Input: part model. Units: mm. Frame: model coordinates. A direction names the side the tool comes from. Round coordinates to 2 decimals unless told otherwise and drop trailing zeros. Loops run counter-clockwise (first coordinate to the right, second up) from the corner with the lowest first, then second, coordinate; pieces in that order, holes last. Notation, with made-up numbers: (-27.75, -28.5) -> (-3.75, -28.5) arc R33 cw to (-3.75, 7.5) -> close; hole circle Ø7 at (69, 74). An arc over 180 degrees is marked (long way). One line per question, with ' | ' between items. Start each with the question number.
Q1. Cut plane B-B on x = -32.5. Return loops of the section in (y, z).
Q2. Cut plane C-C on x = -21. Return loops of the section in (y, z).
Q3. Contact query for flat-ended pins moving along their axis: P1, Ø5.5, axis at x = -29.5, z = -3.5, coming from the +Y side; P2, Ø2.5, axis at x = -11, y = -3, coming from the +Z side; P3, Ø5, axis at x = -9, y = 1.5, coming from the -Z side. Output: stop coordinate, or through.
Q4. Mould query, pull axis Y, two halves, no side actions, for faces 4 (the face through (-6.23, 3.23, -4.55)), 5 (the face through (-47.17, -5.96, 0.02)), 6 (the face through (-47.728, 4.148, 4.897)). Classes: pulls with the +Y half, pulls with the -Y half, needs draft (parallel to the pull), parting line crosses it, or undercut.
Q5. Access query for faces 1 (the face through (-25, 10.058, 5)), 2 (the face through (-4.981, -2.624, -4.55)), 3 (the face through (-4.981, -2.624, 4.65)). Directions: +Z, -Z, +X, -X, +Y, -Y. A direction counts if a zero-diameter tool reaches every point of the face in a straight line with its end or side. Return the directions, or none.
Q6. Material intervals for L1, parallel to X at y = 5.5, z = 4; L2, parallel to X at y = 4.75, z = 5.75; L3, parallel to Z at x = -17, y = 10.5, sorted ascending.
Q7. Cut plane A-A on y = 4.75. Return loops of the section in (x, z), and give its area (3 significant figures).
from build123d import *

# Parameters (mm, degrees)
F1_DEPTH    = 8.2
F2_DEPTH    = 1
F4_DEPTH    = 5.5
F15_DEPTH   = 5.5
F5_R        = 2
F16_R       = 0.5
F17_R       = 2
F18_R       = 5
F19_R       = 0.5
F6_R        = 0.59999
F8_DEPTH    = 8.2
F9_T1_DEPTH = 31.0823571676
F10_R       = 4
F12_DEPTH   = 1.5
F13_R       = 7


# Not quite as in the source:
# - a fillet or chamfer that OpenCascade refuses, or shapes differently, is made with other operations: its cross-section is extruded or revolved along the edge and cut away or added
# - a fillet or chamfer is up to 0.001 mm smaller than in the source, because OpenCascade refuses the exact size


with BuildPart() as f1:
    # F0 (on Top) → F1 (new body, symmetric)
    with BuildSketch(Plane.XY):
        with BuildLine():
            Line((-7.6991717756, 9.5581562555), (-40.1991717756, 9.5581562555))
            ThreePointArc((-40.1991717756, 9.5581562555), (-47.4491717756, 2.3081562555), (-40.1991717756, -4.9418437445))
            ThreePointArc((-40.1991717756, -4.9418437445), (-38.6431985652, -1.6852820196), (-42.1543481568, -2.5207911129))
            ThreePointArc((-42.1543481568, -2.5207911129), (-44.8427156809, 2.8081562555), (-40.1991717756, 6.5581562555))
            Line((-40.1991717756, 6.5581562555), (-16.7462805126, 6.5581562555))
            Line((-16.7462805126, 6.5581562555), (-11.035484998, -2.9462035475))
            ThreePointArc((-11.035484998, -2.9462035475), (-4.6547300014, -4.5371044474), (-3.0638291014, 1.8436505492))
            Line((-3.0638291014, 1.8436505492), (-7.6991717756, 9.5581562555))
        make_face()
        with BuildLine():
            Line((-15.346320436, 6.5581562555), (-8.229856713, 6.5581562555))
            Line((-8.229856713, 6.5581562555), (-4.7781637028, 0.8135743994))
            ThreePointArc((-4.7781637028, 0.8135743994), (-5.8216578415, -3.3716519963), (-10.0068842371, -2.3281578576))
            Line((-10.0068842371, -2.3281578576), (-15.346320436, 6.5581562555))
        make_face(mode=Mode.SUBTRACT)
    extrude(amount=F1_DEPTH, both=True)

    # F0 (on Top) → F2 (join, symmetric)
    with BuildSketch(Plane.XY):
        with BuildLine():
            Line((-4.7781637028, 0.8135743994), (-8.229856713, 6.5581562555))
            Line((-8.229856713, 6.5581562555), (-15.346320436, 6.5581562555))
            Line((-15.346320436, 6.5581562555), (-10.0068842371, -2.3281578576))
            ThreePointArc((-10.0068842371, -2.3281578576), (-5.8216578415, -3.3716519963), (-4.7781637028, 0.8135743994))
        make_face()
    extrude(amount=F2_DEPTH, both=True)

    # F3 (on face) → F4 (cut)
    with BuildSketch(Plane.XY.offset(8.2)):
        Polygon((-9.8084988335, -7.0643632576), (-7.0496570497, -0.5512764992), (-8.3826289276, 1.6671612479), (-13.2850058391, -1.2784839779), align=None)
    extrude(amount=-F4_DEPTH, mode=Mode.SUBTRACT)

    # F14 (on face) → F15 (cut)
    with BuildSketch(Plane(origin=(0, 0, -8.2), x_dir=(1, 0, 0), z_dir=(0, 0, -1))):
        with BuildLine():
            Line((-12.3684568759, 0.7277658005), (-11.3398561151, 0.1097201106))
            Line((-11.3398561151, 0.1097201106), (-10.0068842371, 2.3281578576))
            ThreePointArc((-10.0068842371, 2.3281578576), (-9.3022346771, 3.1354223006), (-8.3618696665, 3.649154264))
            Line((-8.3618696665, 3.649154264), (-8.8633257373, 4.8329941325))
            ThreePointArc((-8.8633257373, 4.8329941325), (-10.099006978, 4.0618270279), (-11.035484998, 2.9462035475))
            Line((-11.035484998, 2.9462035475), (-12.3684568759, 0.7277658005))
        make_face()
    extrude(amount=-F15_DEPTH, mode=Mode.SUBTRACT)

    # F5
    f5_edges = [f1.edges().sort_by_distance(p)[0] for p in [
        (-16.746281, 6.558156, 0),
    ]]
    fillet(f5_edges, radius=F5_R)

    # F16
    f16_edges = [f1.edges().sort_by_distance(p)[0] for p in [
        (-15.34632, 6.558156, -4.6),
        (-15.34632, 6.558156, 4.6),
    ]]
    fillet(f16_edges, radius=F16_R)

    # F17
    f17_edges = [f1.edges().sort_by_distance(p)[0] for p in [
        (-8.229857, 6.558156, -4.6),
        (-8.229857, 6.558156, 4.6),
    ]]
    fillet(f17_edges, radius=F17_R)

    # F18
    f18_edges = [f1.edges().sort_by_distance(p)[0] for p in [
        (-7.699172, 9.558156, 0),
    ]]
    fillet(f18_edges, radius=F18_R)

    # F19
    f19_edges = [f1.edges().sort_by_distance(p)[0] for p in [
        (-42.154348, -2.520791, 0),
    ]]
    fillet(f19_edges, radius=F19_R)

    # F6 (radius 0.6 in the source; OpenCascade refuses exactly that, so slightly less here)
    f6_edges = [f1.edges().sort_by_distance(p)[0] for p in [
        (-12.368457, -0.727766, 5.45),
        (-11.339856, -0.10972, 5.45),
        (-8.36187, -3.649154, 5.45),
        (-8.863326, -4.832994, 5.45),
        (-8.863326, -4.832994, -5.45),
        (-8.36187, -3.649154, -5.45),
        (-12.368457, -0.727766, -5.45),
        (-11.339856, -0.10972, -5.45),
    ]]
    fillet(f6_edges, radius=F6_R)

    # F7 (on Top) → F8 (join, symmetric)
    with BuildSketch(Plane.XY):
        with BuildLine():
            ThreePointArc((-40.1991717756, -4.9418437445), (-47.4491717756, 2.3081562555), (-40.1991717756, 9.5581562555))
            Line((-40.1991717756, 9.5581562555), (-10.5280356666, 9.5581562555))
            ThreePointArc((-10.5280356666, 9.5581562555), (-8.065917866, 8.9099347352), (-6.242199163, 7.13334663))
            Line((-6.242199163, 7.13334663), (-3.0638291014, 1.8436505492))
            ThreePointArc((-3.0638291014, 1.8436505492), (-3.0131583432, -2.8597777863), (-7.0927569488, -5.2010767528))
            Line((-7.0927569488, -5.2010767528), (-4.8792576743, -5.2215941063))
            ThreePointArc((-4.8792576743, -5.2215941063), (-2.1256697511, -2.0601996528), (-2.6352454511, 2.1011695866))
            Line((-2.6352454511, 2.1011695866), (-5.8136155127, 7.3908656675))
            ThreePointArc((-5.8136155127, 7.3908656675), (-7.819706086, 9.3451125832), (-10.5280356666, 10.0581562555))
            Line((-10.5280356666, 10.0581562555), (-40.1991717756, 10.0581562555))
            ThreePointArc((-40.1991717756, 10.0581562555), (-47.9456545804, 2.5416175049), (-40.6658823702, -5.4277781561))
            Line((-40.6658823702, -5.4277781561), (-39.2876185276, -4.7220321267))
            ThreePointArc((-39.2876185276, -4.7220321267), (-39.7303310587, -4.8861144001), (-40.1991717756, -4.9418437445))
        make_face()
    extrude(amount=F8_DEPTH, both=True)

    # F9: fillet of radius 5 on 1 edges, made by hand

    # F9_s2 → F9_t1 (cut)
    with BuildSketch(Plane.XY.offset(-15.5411785838)):
        with BuildLine():
            ThreePointArc((-39.2876185276, -4.7220321267), (-41.4015983231, -5.1781218435), (-43.5104409693, -4.6988399859))
            Line((-43.5104409693, -4.6988399859), (-43.5531670234, -4.7892528406))
            ThreePointArc((-43.5531670234, -4.7892528406), (-42.1478250371, -5.2961353267), (-40.6719044424, -5.5275966647))
            Line((-40.6719044424, -5.5275966647), (-40.6203047078, -5.5167875752))
            ThreePointArc((-40.6203047078, -5.5167875752), (-39.9311727865, -5.1639145605), (-39.2458881329, -4.8129088242))
            Line((-39.2458881329, -4.8129088242), (-39.2876185276, -4.7220321267))
        make_face()
    extrude(amount=F9_T1_DEPTH, mode=Mode.SUBTRACT)

    # F10
    f10_edges = [f1.edges().sort_by_distance(p)[0] for p in [
        (-4.879258, -5.221594, 0),
    ]]
    fillet(f10_edges, radius=F10_R)

    # F11 (on Top) → F12 (join, symmetric)
    with BuildSketch(Plane.XY):
        with BuildLine():
            Line((-9.8019854711, 10.0100230104), (-40.1991717756, 14.0581562555))
            ThreePointArc((-40.1991717756, 14.0581562555), (-51.5354352526, 5.3987274618), (-46.1626661567, -7.8160343179))
            Line((-46.1626661567, -7.8160343179), (-39.3222752617, -4.7377869483))
            ThreePointArc((-39.3222752617, -4.7377869483), (-41.4206326973, -5.1779810716), (-43.5104409693, -4.6988399859))
            ThreePointArc((-43.5104409693, -4.6988399859), (-47.7611398022, 4.0049590032), (-40.1991717756, 10.0581562555))
            Line((-40.1991717756, 10.0581562555), (-10.5280356666, 10.0581562555))
            ThreePointArc((-10.5280356666, 10.0581562555), (-10.1642136992, 10.0461097517), (-9.8019854711, 10.0100230104))
        make_face()
    extrude(amount=F12_DEPTH, both=True)

    # F13
    f13_edges = [f1.edges().sort_by_distance(p)[0] for p in [
        (-46.162666, -7.816034, 0),
    ]]
    fillet(f13_edges, radius=F13_R)


solid = f1.part
Results:
1) outline: (6.56, -8.2) -> (10.06, -8.2) -> (10.06, -1.5) -> (13.03, -1.5) -> (13.03, 1.5) -> (10.06, 1.5) -> (10.06, 8.2) -> (6.56, 8.2) -> close
2) outline: (6.56, -8.2) -> (10.06, -8.2) -> (10.06, -1.5) -> (11.5, -1.5) -> (11.5, 1.5) -> (10.06, 1.5) -> (10.06, 8.2) -> (6.56, 8.2) -> close
3) P1: y = 12.88 | P2: z = 2.7 | P3: z = -1
4) face 4: undercut | face 5: pulls with the -Y half | face 6: parting line crosses it
5) face 1: +Z, +X, -X, +Y | face 2: -Z | face 3: +Z
6) L1: -47.26 to -43.19, -16.11 to -14.71, -7.59 to -4.68 | L2: -47.55 to -43.93, -15.66 to -14.26, -7.14 to -4.23 | L3: -1.5 to 1.5
7) outline: (-51.69, -1.5) -> (-47.55, -1.5) -> (-47.55, -8.2) -> (-43.93, -8.2) -> (-43.93, 8.2) -> (-47.55, 8.2) -> (-47.55, 1.5) -> (-51.69, 1.5) -> close; (-15.66, -8.2) -> (-14.26, -8.2) -> (-14.26, -1) -> (-7.14, -1) -> (-7.14, -8.2) -> (-4.23, -8.2) -> (-4.23, 8.2) -> (-7.14, 8.2) -> (-7.14, 1) -> (-14.26, 1) -> (-14.26, 8.2) -> (-15.66, 8.2) -> close | area: 157 mm^2
